```python
from build123d import *

# Parameters (mm, degrees)
BOSS_EXTRUDE1_DEPTH      = 4
BOSS_EXTRUDE2_DEPTH      = 4
BOSS_EXTRUDE2_DEPTH_BACK = 12.7
CUT_EXTRUDE1_START       = -8
SKETCH2_R                = 4.15
CUT_EXTRUDE1_DEPTH       = 5.95
SKETCH3_R                = 1.6
CUT_EXTRUDE2_DEPTH       = 32.16390509


with BuildPart() as part:
    # Sketch1 → Boss-Extrude1 (new, symmetric)
    with BuildSketch(Plane(origin=(0, 0, 0), x_dir=(1, 0, 0), z_dir=(0, 1, 0))):
        with BuildLine():
            ThreePointArc((6.498753649, 0.127283164), (-1.682323793, 6.278517871), (-5.691727336, -3.139146371))
            ThreePointArc((-5.691727336, -3.139146371), (1.620767152, -6.294689336), (6.5, 0))
            ThreePointArc((6.5, 0), (6.499688405, 0.063644633), (6.498753649, 0.127283164))
        make_face()
        with BuildLine():
            ThreePointArc((6.5, 0), (1.620767152, -6.294689336), (-5.691727336, -3.139146371))
            Line((-5.691727336, -3.139146371), (2.048950522, -17.174117205))
            ThreePointArc((2.048950522, -17.174117205), (4.906448368, -18.407206302), (6.813102435, -15.947435392))
            ThreePointArc((6.813102435, -15.947435392), (6.812980673, -15.922565028), (6.812615399, -15.897697048))
            Line((6.812615399, -15.897697048), (6.563875983, -3.197697048))
            Line((6.563875983, -3.197697048), (6.498753649, 0.127283164))
            ThreePointArc((6.498753649, 0.127283164), (6.499688405, 0.063644633), (6.5, 0))
        make_face()
        with BuildLine():
            ThreePointArc((6.812615399, -15.897697048), (6.812980673, -15.922565028), (6.813102435, -15.947435392))
            Line((6.813102435, -15.947435392), (6.813102435, -3.197697048))
            Line((6.813102435, -3.197697048), (6.563875983, -3.197697048))
            Line((6.563875983, -3.197697048), (6.812615399, -15.897697048))
        make_face()
        with BuildLine():
            ThreePointArc((6.813102435, -15.947435392), (4.906448368, -18.407206302), (2.048950522, -17.174117205))
            Line((2.048950522, -17.174117205), (6.813102435, -25.812215104))
            Line((6.813102435, -25.812215104), (6.813102435, -15.947435392))
        make_face()
    extrude(amount=BOSS_EXTRUDE1_DEPTH, both=True)

    # Sketch1<3> → Boss-Extrude2 (add, two sides: drawn at the far end of the back side and taken through both)
    with BuildSketch(Plane(origin=(0, 0, 0), x_dir=(1, 0, 0), z_dir=(0, 1, 0)).offset(-BOSS_EXTRUDE2_DEPTH_BACK)):
        Polygon((6.813102435, -15.947435392), (6.813102435, -25.812215104), (6.813102435, -28.597697048), (8.813098435, -28.597697048), (8.813098435, -3.197697048), (6.813102435, -3.197697048), align=None)
    extrude(amount=BOSS_EXTRUDE2_DEPTH + BOSS_EXTRUDE2_DEPTH_BACK)

    # Sketch2 → Cut-Extrude1 (cut)
    with BuildSketch(Plane.XZ.offset(4).offset(CUT_EXTRUDE1_START)):
        with Locations(Location((0, 0, 0), (0, 0, 90))):
            Circle(SKETCH2_R)
    extrude(amount=CUT_EXTRUDE1_DEPTH, mode=Mode.SUBTRACT)

    # Sketch3 → Cut-Extrude2 (cut, through all)
    with BuildSketch(Plane.XZ.offset(4)):
        with Locations(Location((0, 0, 0), (0, 0, 270))):
            Circle(SKETCH3_R)
    extrude(amount=-CUT_EXTRUDE2_DEPTH, mode=Mode.SUBTRACT)


solid = part.part
```
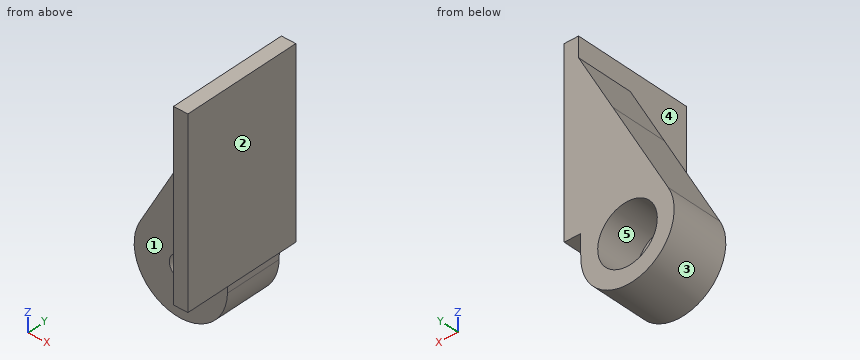
Can you work these out from the model? Positions are in its coordinate system, mm. Face numbers are marked on the shaded views. A direction names the side the tool comes from. Give positions to 0.01 mm unless a question says otherwise; leave off trailing zeros. Loops run counter-clockwise (first coordinate to the right, second up) from the corner with the lowest first, then second, coordinate; pieces in that order, holes last. Notation, with made-up numbers: M 60.25,-29.5 L 106.25,-29.5 A23 cw 106.25,-9.5 Z; hole C -29.75,46.25 d8. An arc over 180 degrees is marked long. One line per question, with ' | ' between items. Start each with the question number.
Q1. If we section it at C-C (z = 26.5): Please give me the cut outline in (x, y), plus the area to 3 significant figures.
Q2. If I drill on line 1 (X direction, y = 1.95, z = 0); line 2 (X direction, y = -4.5, z = 9); line 3 (Y direction, x = 5, z = 19), over which ranges is the centre line in solid material (lowest first)? Write a range as from..to.
Q3. If we section it at B-B (z = 0.5): Please give me the cut outline in (x, y), plus the area to 3 significant figures.
Q4. If we mould it in two halves opening along Z, with no side actions, what happens to the marked faces 3, 4 and 5? For each: +Z half, -Z half, draft (parallel to the pull), parting line (faces both ways), or undercut.
Q5. If we section it at D-D (y = -10): Please give me the cut outline in (x, z).
Q6. For the marked faces 1 and 2, which set-ups out of +Z, -Z, +X, -X, +Y, -Y let a thin tool reach every point of the face, with its end or its side?
Q7. For pin 1 Ø3.5 at (x, z) = (0, 0) entering from -Y; pin 2 Ø2.5 at (x, z) = (1.5, 1.5) entering from +Y; pin 3 Ø8.5 at (y, z) = (-4, 11.5) entering from -X; pin 4 Ø3 at (x, y) = (-2.5, -6) entering from +Z (3 decimals), each with a flat end and sliding along its axis, tell me the tip position at first contact or that it passes through.
Q8. If we section it at A-A (x = 0): Please give me the cut outline in (y, z), plus the area to 3 significant figures.
Computed:
1) outline: M 6.81,-12.7 L 8.81,-12.7 L 8.81,4 L 6.81,4 Z | area: 33.4 mm²
2) line 1: x = -6.5..-4.15, 4.15..6.5 | line 2: x = 6.81..8.81 | line 3: y = -4..4
3) outline: M -6.48,-4 L -1.52,-4 L -1.52,-1.95 L -4.12,-1.95 L -4.12,4 L -6.48,4 Z; M 1.52,-4 L 6.51,-4 L 6.51,4 L 4.12,4 L 4.12,-1.95 L 1.52,-1.95 Z | area: 48.7 mm²
4) face 3: parting line | face 4: draft | face 5: undercut
5) outline: M 6.81,3.2 L 8.81,3.2 L 8.81,28.6 L 6.81,28.6 Z
6) face 1: +Z, -Z, -X, -Y | face 2: +Z, -Z, +X, +Y, -Y
7) pin 1: stops at y = -4 | pin 2: stops at y = -1.95 | pin 3: stops at x = -3.42 | pin 4: passes through
8) outline: M -4,-6.5 L 4,-6.5 L 4,-4.15 L -1.95,-4.15 L -1.95,-1.6 L -4,-1.6 Z; M -4,1.6 L -1.95,1.6 L -1.95,4.15 L 4,4.15 L 4,13.46 L -4,13.46 Z | area: 104 mm²
